Could you check a few things on this model? Use its own coordinates, in mm. Give positions to 0.01 mm unless a question says otherwise; leave off trailing zeros. Write each loop counter-clockwise with the first axis right and the second up, starting at its lowest first coordinate (ties: lowest second). Pieces come first, ordered by that corner, then holes. Notation, with made-up numbers: (-24, 83) - (-1, 83) arc R11 cw to (-1, 88) - close; hole circle Ø5 at (-26, 28.25). An arc over 180 degrees is marked (long way). Write item = value, one per line.
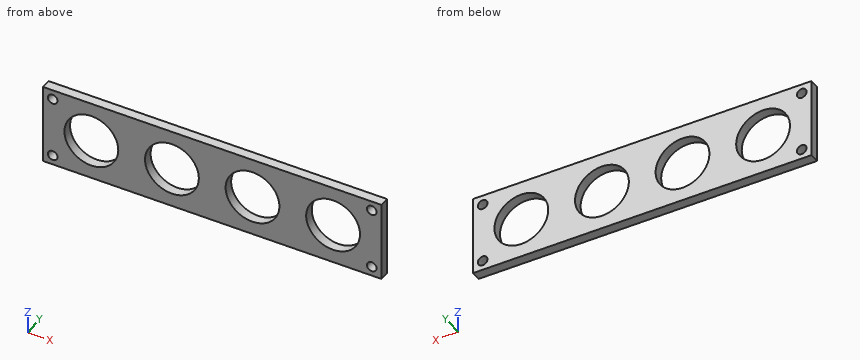
from build123d import *

# Parameters (mm, degrees)
F0_R     = 1.5
F0_R_2   = 8.35
F1_DEPTH = 3


with BuildPart() as f1:
    # F0 (on Front) → F1 (new body)
    with BuildSketch(Plane.XZ):
        Polygon((-48.303484, 6.842105), (-48.303484, -5.657895), (56.696516, -5.657895), (56.696516, 6.842105), (56.696516, 19.342105), (-48.303484, 19.342105), align=None)
        with Locations((-45.303484, -2.657895)):
            Circle(F0_R, mode=Mode.SUBTRACT)
        with Locations((-33.303484, 6.842105)):
            Circle(F0_R_2, mode=Mode.SUBTRACT)
        with Locations((-8.303484, 6.842105)):
            Circle(F0_R_2, mode=Mode.SUBTRACT)
        with Locations((53.696516, -2.657895)):
            Circle(F0_R, mode=Mode.SUBTRACT)
        with Locations((16.696516, 6.842105)):
            Circle(F0_R_2, mode=Mode.SUBTRACT)
        with Locations((41.696516, 6.842105)):
            Circle(F0_R_2, mode=Mode.SUBTRACT)
        with Locations((-45.303484, 16.342105)):
            Circle(F0_R, mode=Mode.SUBTRACT)
        with Locations((53.696516, 16.342105)):
            Circle(F0_R, mode=Mode.SUBTRACT)
    extrude(amount=F1_DEPTH)


solid = f1.part
1. I need wall thicknesses on line 1 (X direction, y = -2.7, z = 16.25); line 2 (X direction, y = -0.4, z = 8.5); line 3 (X direction, y = -0.45, z = 9.75). Which ranges of each line are inside material? Lowest first, please.
Filled sheet:
line_1 = -48.3 to -46.8, -43.81 to 52.2, 55.19 to 56.7
line_2 = -48.3 to -41.49, -25.12 to -16.49, -0.12 to 8.51, 24.88 to 33.51, 49.88 to 56.7
line_3 = -48.3 to -41.13, -25.48 to -16.13, -0.48 to 8.87, 24.52 to 33.87, 49.52 to 56.7
2. If we section it at D-D, the plane z = 5.75: Please give me the cut outline in (x, y), and give its area (3 significant figures).
Filled sheet:
outline = (-48.3, -3) - (-41.58, -3) - (-41.58, 0) - (-48.3, 0) - close; (-25.03, -3) - (-16.58, -3) - (-16.58, 0) - (-25.03, 0) - close; (-0.03, -3) - (8.42, -3) - (8.42, 0) - (-0.03, 0) - close; (24.97, -3) - (33.42, -3) - (33.42, 0) - (24.97, 0) - close; (49.97, -3) - (56.7, -3) - (56.7, 0) - (49.97, 0) - close
area = 116 mm2
3. If we section it at C-C, the plane y = -2.05: Count the separate pieces of the cut face and the enclosed holes in it, and give its area (3 significant figures).
Filled sheet:
separate_pieces = 1
enclosed_holes = 8
area = 1,720 mm2
4. If we section it at B-B, the plane x = 36.5: Please give me the cut outline in (y, z), and give its area (3 significant figures).
Filled sheet:
outline = (-3, -5.66) - (0, -5.66) - (0, 0.31) - (-3, 0.31) - close; (-3, 13.38) - (0, 13.38) - (0, 19.34) - (-3, 19.34) - close
area = 35.8 mm2
5. For pin 1 (1.8 mm diameter, centred on x = -45.3, z = 16.34, fed in from +Y), with a flat end and sliding along its axis, tell me the tip position at first contact or that it passes through.
Filled sheet:
pin_1 = through
6. If we section it at A-A, the plane z = 1: Please give me the cut outline in (x, y), and give its area (3 significant figures).
Filled sheet:
outline = (-48.3, -3) - (-39.27, -3) - (-39.27, 0) - (-48.3, 0) - close; (-27.34, -3) - (-14.27, -3) - (-14.27, 0) - (-27.34, 0) - close; (-2.34, -3) - (10.73, -3) - (10.73, 0) - (-2.34, 0) - close; (22.66, -3) - (35.73, -3) - (35.73, 0) - (22.66, 0) - close; (47.66, -3) - (56.7, -3) - (56.7, 0) - (47.66, 0) - close
area = 172 mm2
